Read the model definition and answer for the solid it produces. Units are mm, in the model's axes. A direction names the side the tool comes from. Give positions to 0.01 mm unless a question says otherwise; leave off trailing zeros. Write each loop counter-clockwise with the first axis right and the second up, starting at its lowest first coordinate (ties: lowest second). Pieces come first, ordered by that corner, then holes.
Autodesk Fusion 360 part; units mm, degrees
sketch "Tool" plane through (0, 0, 0) normal (0, 0, 1) x (1, 0, 0)
  circle A0 centre (0, 0) radius 10.415
  circle A1 centre (0, 0) radius 9.6
  line L0 (-10.415, 0.0013) -> (10.415, 0.0013) construction
  line L1 (0, 10.485) -> (0, -10.415) construction
  line L2 (-10.415, -0.7737) -> (10.415, -0.7737)
  line L3 (-10.415, 0.7763) -> (10.415, 0.7763)
  line L4 (-0.775, 10.485) -> (-0.775, -10.415)
  line L5 (0.775, 10.485) -> (0.775, -10.415)
  circle A2 centre (0, 0) radius 11.415
  dimension "d5" = 20.83
  dimension "d6" = 19.2
  dimension "d7" = 0.775
  dimension "d8" = -0.775
  dimension "d9" = 0.775
  dimension "d10" = -0.775
  dimension "d13" = 1
extrude "Extrude1" add sketch "Tool" against normal blind 8 contours A0 A1 L2 L3 | A0 A1 L4 L5 | A0 A1 L4 L5 | A0 A1 L2 L3 | A2
move_face "OffsetFaces1" offset -0.05 17 faces at (10.7291, 0.0008, 0) (1.7545, 10.2662, -5.3333) (9.5903, 0.4322, -2.6667) (8.0289, -6.6339, -5.3333) (9.8411, 0.7763, -2.6667) (9.8413, -0.7737, -2.6667) (0.775, 10.1136, -5.3333) (-0.603, 9.581, -5.3333) (-7.0069, 7.7056, -5.3333) (-10.1137, -0.7737, -2.6667) (-0.775, 10.1136, -2.6667) (0.775, -9.8412, -5.3333) (0.603, -9.581, -5.3333) (-1.2662, -10.3377, -5.3333) (-9.5904, -0.4296, -5.3333) (-0.775, -9.8412, -2.6667) (-10.1135, 0.7763, -2.6667)
sketch "Sketch2" plane through (0, 0, -0.05) normal (0, 0, 1) x (-1, 0, 0)
  arc A0 (-9.6228, 0.7237) -> (-9.6226, -0.7263) centre (0, 0) ccw
  line L0 (-9.6228, 0.7237) -> (-10.4399, 0.7237)
  arc A1 (-0.725, 10.4399) -> (-10.4399, 0.7237) centre (0, 0) ccw
  line L1 (-0.725, 10.4399) -> (-0.725, 9.6227)
  arc A2 (0.725, 9.6227) -> (-0.725, 9.6227) centre (0, 0) ccw
  line L2 (0.725, 9.6227) -> (0.725, 10.4399)
  arc A3 (10.4399, 0.7237) -> (0.725, 10.4399) centre (0, 0) ccw
  line L3 (10.4399, 0.7237) -> (9.6228, 0.7237)
  arc A4 (9.6226, -0.7263) -> (9.6228, 0.7237) centre (0, 0) ccw
  line L4 (9.6226, -0.7263) -> (10.4398, -0.7263)
  arc A5 (0.725, -10.4399) -> (10.4398, -0.7263) centre (0, 0) ccw
  line L5 (0.725, -10.4399) -> (0.725, -9.6227)
  arc A6 (-0.725, -9.6227) -> (0.725, -9.6227) centre (0, 0) ccw
  line L6 (-0.725, -9.6227) -> (-0.725, -10.4399)
  arc A7 (-10.4398, -0.7263) -> (-0.725, -10.4399) centre (0, 0) ccw
  line L7 (-10.4398, -0.7263) -> (-9.6226, -0.7263)
  circle A8 centre (0, 0) radius 11.415
  line L8 (0, 0) -> (8.0716, -8.0716) construction
  line L9 (0, 0) -> (11.415, 0) construction
  line L10 (0, 0) -> (8.0716, 8.0716) construction
  line L11 (0, 0) -> (11.415, 0) construction
  line L12 (0, 0) -> (-8.0716, -8.0716) construction
  line L13 (0, 0) -> (-8.0716, 8.0716) construction
  line L14 (0.7071, 0.7071) -> (8.7787, -7.3645)
  line L15 (0.7071, 0.7071) -> (-7.3645, 8.7787)
  line L16 (-0.7071, -0.7071) -> (-8.7787, 7.3645)
  line L17 (-0.7071, -0.7071) -> (7.3645, -8.7787)
  line L18 (0.7071, -0.7071) -> (8.7787, 7.3645)
  line L19 (0.7071, -0.7071) -> (-7.3645, -8.7787)
  line L20 (-0.7071, 0.7071) -> (7.3645, 8.7787)
  line L21 (-0.7071, 0.7071) -> (-8.7787, -7.3645)
  dimension "d17" = 45
  dimension "d18" = 45
  dimension "d19" = 90
  dimension "d20" = 1
  dimension "d21" = -1
  dimension "d22" = 1
  dimension "d23" = -1
extrude "Extrude2" add sketch "Sketch2" along normal blind 8 and the other way blind 2 contours A1 A8 L15 L16 | A1 L15 L16 L20 L21 | A7 L16 L17 L19 L21 | A7 A8 L19 L21 | L14 L15 L16 L17 L18 L19 L20 L21 | A3 L14 L15 L18 L20 | A5 L14 L17 L18 L19 | A3 A8 L18 L20 | A5 A8 L14 L17
extrude "Extrude3" add sketch "Tool" along normal blind 8
equation "outside_diamter = 20.83 mm"
equation "wall_thickness = 1.63 mm"
equation "tool_teeth_width = 1.55 mm"
equation "inside_diamter = outside_diamter - wall_thickness"
equation "d5 = outside_diamter"
equation "d6 = inside_diamter"
equation "d7 = tool_teeth_width / 2"
equation "d8 = -( tool_teeth_width / 2 )"
equation "d9 = tool_teeth_width / 2"
equation "d10 = -( tool_teeth_width / 2 )"
equation "tool_thickness = 1 mm"
equation "tool_depth = 8 mm"
equation "d13 = tool_thickness"
Item 1: Find the intervals of material crossed by line 1 along Y through (x, z) = (-6, 3.75); line 2 along Y through (x, z) = (4.5, 5); line 3 along X through (y, z) = (-2, 6.25), in increasing order.
Result set:
line 1: y = -9.71 to -8.51, -7.41 to -4.59, 4.59 to 7.41, 8.51 to 9.71
line 2: y = -10.49 to -9.39, -5.91 to -3.09, 3.09 to 5.91, 9.39 to 10.49
line 3: x = -11.24 to -10.22, -3.41 to -0.59, 0.59 to 3.41, 10.22 to 11.24
Item 2: Section C-C (y = 7) is taken. Write down the section's boundary in (x, z), and give its area (3 significant figures).
Result set:
outline: (-9.02, -8) - (-7.78, -8) - (-7.78, -2.05) - (-5.59, -2.05) - (-5.59, 7.95) - (-7.71, 7.95) - (-7.71, 8) - (-9.02, 8) - (-9.02, 0) - (-8.41, 0) - (-8.41, -0.05) - (-9.02, -0.05) - close; (5.59, -2.05) - (7.78, -2.05) - (7.78, -8) - (9.02, -8) - (9.02, -0.05) - (8.41, -0.05) - (8.41, 0) - (9.02, 0) - (9.02, 8) - (7.71, 8) - (7.71, 7.95) - (5.59, 7.95) - close
area: 83.4 mm2
Item 3: Section B-B (y = 4) is taken. Write down the section's boundary in (x, z).
Result set:
outline: (-10.69, -8) - (-9.67, -8) - (-9.67, -0.05) - (-10.69, -0.05) - close; (-10.69, 0) - (-9.62, 0) - (-9.62, 8) - (-10.69, 8) - close; (-5.41, -2.05) - (-2.59, -2.05) - (-2.59, 7.95) - (-5.41, 7.95) - close; (2.59, -2.05) - (5.41, -2.05) - (5.41, 7.95) - (2.59, 7.95) - close; (9.62, 0) - (10.69, 0) - (10.69, 8) - (9.62, 8) - close; (9.67, -8) - (10.69, -8) - (10.69, -0.05) - (9.67, -0.05) - close
Item 4: Section D-D (z = -1.25) is taken. Give the number of separate pieces and of enclosed holes in the cut face, and give its area (3 significant figures).
Result set:
separate pieces: 1
enclosed holes: 4
area: 150 mm2
Item 5: Each of these flat-tipped pins is pushed along its axis until it touches: pin 1 Ø2 at (y, z) = (-6, 0.5) entering from +X; pin 2 Ø0.7 at (x, z) = (10, -4) entering from -Y; pin 3 Ø1 at (y, z) = (-3, -2.5) entering from +X. Where does it stop, or does it pass through?
Result set:
pin 1: stops at x = 10.26
pin 2: stops at y = -6.1
pin 3: stops at x = 11.14
Item 6: Section A-A (z = 6.75) is taken. Write down the section's boundary in (x, y) (1 decimal), and give its area (3 significant figures).
Result set:
outline: circle Ø22.8 at (0, 0); hole (-8, -6.6) - (-1.4, 0) - (-8, 6.6) arc R10.4 ccw to start; hole (-6.6, -8) arc R10.4 ccw to (6.6, -8) - (0, -1.4) - close; hole (-6.6, 8) - (0, 1.4) - (6.6, 8) arc R10.4 ccw to start; hole (1.4, 0) - (8, -6.6) arc R10.4 ccw to (8, 6.6) - close
area: 148 mm2
Item 7: Which of the six approach directions +Z, -Z, +X, -X, +Y, -Y give full straight-line access (tool end or side, diameter ignored) to faces 1 (the flat face through (-10, 0, -0.05)), 2 (the cylindrical face through (0.01, 9.65, -3.97)), 3 (the cylindrical face through (7.5, 7.3, -4))?
Result set:
face 1: -X
face 2: +Z, -Z
face 3: -Z
